Autodesk Inventor part; units mm, degrees
ref_plane "YZ Plane" through (0, 0, 0) normal (1, 0, 0) x (0, 1, 0)
ref_plane "XZ Plane" through (0, 0, 0) normal (0, 1, 0) x (-1, 0, 0)
ref_plane "XY Plane" through (0, 0, 0) normal (0, 0, 1) x (1, 0, 0)
sketch "Esboço1" plane through (0, 0, 0) normal (0, 1, 0) x (-1, 0, 0)
  line L0 (17.5, 32.5) -> (-17.5, 32.5)
  line L1 (-17.5, 32.5) -> (-17.5, -32.5)
  line L2 (-17.5, -32.5) -> (17.5, -32.5)
  line L3 (17.5, -32.5) -> (17.5, 32.5)
  line L4 (17.5, 32.5) -> (-17.5, -32.5) construction
  line L5 (-17.5, 32.5) -> (17.5, -32.5) construction
  point P0 (0, 0)
  dimension "d0" = 35
  dimension "d1" = 65
extrude "Extrusão1" add sketch "Esboço1" along normal blind 10
fillet "Arredondamento1" radius 5 4 edges at (17.5, 5, 32.5) (-17.5, 5, 32.5) (17.5, 5, -32.5) (-17.5, 5, -32.5)
sketch "Esboço2" plane through (-17.5, 0, -27.5) normal (-1, 0, 0) x (0, 0, 1)
  line L0 (16.5, -3) -> (38.5, -3)
  line L1 (38.5, -3) -> (38.5, 3)
  line L2 (38.5, 3) -> (16.5, 3)
  line L3 (16.5, 3) -> (16.5, -3)
  line L4 (16.5, -3) -> (38.5, 3) construction
  line L5 (38.5, -3) -> (16.5, 3) construction
  point P0 (27.5, 0)
  dimension "d5" = 22
  dimension "d6" = 6
extrude "Extrusão2" cut sketch "Esboço2" against normal up to surface (35 mm away)
properties part number "ESC BASE"
Geometry check sheet. Reference: the model listing, model coordinates, mm. A direction names the side the tool comes from. Coordinates: 2 decimals unless noted, no trailing zeros. Order: outer loops, then holes, each group sorted by start corner. A loop starts at its lowest first (then second) coordinate and runs counter-clockwise, first axis right, second up. Notation, with made-up numbers: M -23.5,60 L 31.5,60 A29 ccw 31.5,81 Z; hole C 7,32.5 d3. An arc over 180 degrees is marked long. One line per question, with ' | ' between items. Start each with the question number.
Item 1: Set-up check for faces 4 (the flat face through (-17.5, 5, 0)), 5 (the flat face through (0, 2, -11)): record each of +Z, -Z, +X, -X, +Y, -Y from which the full face is reachable in a straight line by a thin tool's end or side.
Item 2: Cross-section at C-C on z = -9. Enter the section's corners in (x, y).
Item 3: Cross-section at D-D on x = 14.5. Enter the section's corners in (y, z), then the cut area to 3 significant figures.
Item 4: Material ranges on L1, parallel to Z at x = -0.5, y = 2; L2, parallel to Y at x = 15, z = 1; L3, parallel to X at y = 9.5, z = 29, recorded low to high. Write a range as [from, to].
Item 5: Cross-section at B-B on x = -5.5. Enter the section's corners in (y, z).
Item 6: Draft check along Z on faces 1 (the flat face through (0, 1, 11)), 2 (the cylindrical face through (16.07, 5.07, -31)), 3 (the flat face through (0, 0, -22)). Enter one of: pulls with the +Z half, pulls with the -Z half, needs draft (parallel to the pull), parting line crosses it, or undercut.
Item 7: Gauge pin test, flat end, axial feed: pin 1 (6.5 mm diameter, centred on x = 4.5, z = 2, fed in from -Y). Record the tip position at first contact, or that the pin passes through.
Item 8: Cross-section at A-A on y = 2.25. Enter the section's corners in (x, z), then the cut area to 3 significant figures.
Findings:
1) face 4: +Z, -Z, -X, +Y, -Y | face 5: +X, -X, -Y
2) outline: M -17.5,3 L 17.5,3 L 17.5,10 L -17.5,10 Z
3) outline: M 0,-32.08 L 10,-32.08 L 10,32.08 L 0,32.08 L 0,11 L 3,11 L 3,-11 L 0,-11 Z | area: 576 mm²
4) L1: z = [-32.5, -11], [11, 32.5] | L2: y = [3, 10] | L3: x = [-17.27, 17.27]
5) outline: M 0,-32.5 L 10,-32.5 L 10,32.5 L 0,32.5 L 0,11 L 3,11 L 3,-11 L 0,-11 Z
6) face 1: undercut | face 2: pulls with the -Z half | face 3: needs draft
7) pin 1: stops at y = 3
8) outline: M -17.5,-27.5 A5 ccw -12.5,-32.5 L 12.5,-32.5 A5 ccw 17.5,-27.5 L 17.5,-11 L -17.5,-11 Z; M -17.5,11 L 17.5,11 L 17.5,27.5 A5 ccw 12.5,32.5 L -12.5,32.5 A5 ccw -17.5,27.5 Z | area: 1,480 mm²
